```python
from build123d import *

# Parameters (mm, degrees)
F0_W              = 482.6
F0_H              = 1065.2125
F1_DEPTH          = 1.6
F2_W              = 15.875
F2_H              = 1065.2125
F3_DEPTH          = 1.6
F4_W              = 15.875
F4_H              = 1065.2125
F5_DEPTH          = 1.6
F6_W              = 476.25
F6_H              = 15.875
F7_DEPTH          = 1.6
F8_W              = 476.25
F8_H              = 15.875
F9_DEPTH          = 1.6
F10_W             = 381
F10_H             = 963.6125
F11_DEPTH         = 1.6
F12_W             = 3.96875
F12_H             = 6.35
F13_DEPTH         = 1.6
F13_COPIES3_COUNT = 2
F13_COPIES3_PITCH = 1094.309536
F13_COPIES4_COUNT = 2
F13_COPIES4_PITCH = 823.333045
F14_W             = 3.96875
F14_H             = 6.35
F15_DEPTH         = 1.6
F16_W             = 22.225
F16_H             = 12.7
F17_DEPTH         = 16


# Not quite as in the source:
# - a pattern or mirror of a feature is missing from the dataset's text; its kind, count and spacing are read off the source's solid


with BuildPart() as f1:
    # F0 (on Front) → F1 (new body)
    with BuildSketch(Plane.XZ):
        Rectangle(F0_W, F0_H)
    extrude(amount=-F1_DEPTH)

    # F2 (on face) → F3 (join)
    with BuildSketch(Plane(origin=(-241.3, 0, 0), x_dir=(0, -1, 0), z_dir=(-1, 0, 0))):
        with Locations((-7.9375, 0)):
            Rectangle(F2_W, F2_H)
    extrude(amount=-F3_DEPTH)

    # F4 (on face) → F5 (join)
    with BuildSketch(Plane.YZ.offset(241.3)):
        with Locations((7.9375, 0)):
            Rectangle(F4_W, F4_H)
    extrude(amount=-F5_DEPTH)

    # F6 (on face) → F7 (join)
    with BuildSketch(Plane.XY.offset(532.60625)):
        with Locations((0, 7.9375)):
            Rectangle(F6_W, F6_H)
    extrude(amount=-F7_DEPTH)

    # F8 (on face) → F9 (join)
    with BuildSketch(Plane(origin=(0, 0, -532.60625), x_dir=(1, 0, 0), z_dir=(0, 0, -1))):
        with Locations((0, -7.9375)):
            Rectangle(F8_W, F8_H)
    extrude(amount=-F9_DEPTH)

    # F10 (on face) → F11 (cut)
    with BuildSketch(Plane.XZ):
        Rectangle(F10_W, F10_H)
    extrude(amount=-F11_DEPTH, mode=Mode.SUBTRACT)

    # F12 (on face) → F13 (cut)
    with BuildSketch(Plane.XZ):
        with Locations((-232.5, -495.3)):
            Rectangle(F12_W, F12_H)
        with BuildLine():
            Line((-230.515625, -492.125), (-230.515625, -498.475))
            ThreePointArc((-230.515625, -498.475), (-227.340625, -495.3), (-230.515625, -492.125))
        make_face()
        with BuildLine():
            ThreePointArc((-234.484375, -492.125), (-237.659375, -495.3), (-234.484375, -498.475))
            Line((-234.484375, -498.475), (-234.484375, -492.125))
        make_face()
    f13 = extrude(amount=-F13_DEPTH, mode=Mode.SUBTRACT)

    # F13_copies: F13 across plane
    add(f13.mirror(Plane.XY), mode=Mode.SUBTRACT)

    # F13_copies1: F13 across plane
    add(f13.mirror(Plane.XY.offset(-155.575)), mode=Mode.SUBTRACT)

    # F13_copies2: F13 across plane
    add(f13.mirror(Plane(origin=(0, 0, 0), x_dir=(0, 0, 1), z_dir=(1, 0, 0))), mode=Mode.SUBTRACT)

    # F13_copies3: F13 ×2
    with Locations(*[Vector(0.4249254757, 0, 0.9052283359) * (i * F13_COPIES3_PITCH) for i in range(1, F13_COPIES3_COUNT)]):
        add(f13, mode=Mode.SUBTRACT)

    # F13_copies4: F13 ×2
    with Locations(*[Vector(0.5647775259, 0, 0.8252432043) * (i * F13_COPIES4_PITCH) for i in range(1, F13_COPIES4_COUNT)]):
        add(f13, mode=Mode.SUBTRACT)

    # F14 (on face) → F15 (cut)
    with BuildSketch(Plane.XZ):
        with Locations((-232.5, -184.15)):
            Rectangle(F14_W, F14_H)
        with BuildLine():
            Line((-230.515625, -180.975), (-230.515625, -187.325))
            ThreePointArc((-230.515625, -187.325), (-227.340625, -184.15), (-230.515625, -180.975))
        make_face()
        with BuildLine():
            ThreePointArc((-234.484375, -180.975), (-237.659375, -184.15), (-234.484375, -187.325))
            Line((-234.484375, -187.325), (-234.484375, -180.975))
        make_face()
    f15 = extrude(amount=-F15_DEPTH, mode=Mode.SUBTRACT)

    # F15_copies: F15 across plane
    add(f15.mirror(Plane(origin=(0, 0, 0), x_dir=(0, 0, 1), z_dir=(1, 0, 0))), mode=Mode.SUBTRACT)

    # F16 (on face) → F17 (cut)
    with BuildSketch(Plane.XZ):
        with Locations((-230.1875, 515.540625)):
            Rectangle(F16_W, F16_H)
        with BuildLine():
            Line((-219.075, 521.890625), (-219.075, 509.190625))
            ThreePointArc((-219.075, 509.190625), (-212.725, 515.540625), (-219.075, 521.890625))
        make_face()
    extrude(amount=-F17_DEPTH, mode=Mode.SUBTRACT)


solid = f1.part
```
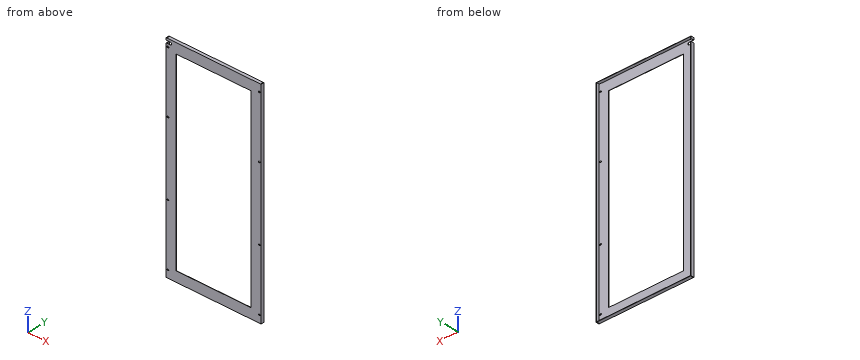
Here's how the part is built. I have some questions about the finished solid (model axes, mm). Coordinates: 2 decimals unless noted, no trailing zeros. Order: outer loops, then holes, each group sorted by start corner. A loop starts at its lowest first (then second) coordinate and runs counter-clockwise, first axis right, second up.
Item 1: If we section it at C-C, the plane z = 273: List the corners of the cut face in (x, y) for me (3 decimals).
Response values:
outline: (-241.3, 0) - (-190.5, 0) - (-190.5, 1.6) - (-239.7, 1.6) - (-239.7, 15.875) - (-241.3, 15.875) - close; (190.5, 0) - (241.3, 0) - (241.3, 15.875) - (239.7, 15.875) - (239.7, 1.6) - (190.5, 1.6) - close
Item 2: If we section it at B-B, the plane y = 9.25: List the corners of the cut face in (x, z) for me (3 decimals).
Response values:
outline: (-241.3, -532.606) - (-239.7, -532.606) - (-239.7, 509.191) - (-241.3, 509.191) - close; (-241.3, 521.891) - (-239.7, 521.891) - (-239.7, 532.606) - (-241.3, 532.606) - close; (-238.125, -532.606) - (238.125, -532.606) - (238.125, -531.006) - (-238.125, -531.006) - close; (-238.125, 531.006) - (238.125, 531.006) - (238.125, 532.606) - (-238.125, 532.606) - close; (239.7, -532.606) - (241.3, -532.606) - (241.3, 532.606) - (239.7, 532.606) - close
Item 3: I need wall thicknesses on probe 1 along X at (y, z) = (6.25, -106); probe 2 along Z at (x, y) = (41.5, 7); probe 3 along Y at (x, z) = (194, -178). Which ranges of each line are inside material? Lowest first, please.
Response values:
probe 1: x = -241.3 to -239.7, 239.7 to 241.3
probe 2: z = -532.61 to -531.01, 531.01 to 532.61
probe 3: y = 0 to 1.6
Item 4: If we section it at A-A, the plane x = 126.5: List the corners of the cut face in (y, z) for me (3 decimals).
Response values:
outline: (0, -532.606) - (15.875, -532.606) - (15.875, -531.006) - (1.6, -531.006) - (1.6, -481.806) - (0, -481.806) - close; (0, 481.806) - (1.6, 481.806) - (1.6, 531.006) - (15.875, 531.006) - (15.875, 532.606) - (0, 532.606) - close
